```python
from build123d import *

# Parameters (mm, degrees)
F0_W     = 110
F0_H     = 55
F1_DEPTH = 60
F3_DEPTH = 60.001
F5_DEPTH = 35


with BuildPart() as f1:
    # F0 (on Top) → F1 (new body)
    with BuildSketch(Plane.XY):
        Rectangle(F0_W, F0_H)
    extrude(amount=F1_DEPTH)

    # F2 (on face) → F3 (cut, through all)
    with BuildSketch(Plane.XY.offset(60)):
        Polygon((-15, -27.5), (-55, 12.5), (-55, -27.5), align=None)
    extrude(amount=-F3_DEPTH, mode=Mode.SUBTRACT)

    # F4 (on face) → F5 (cut)
    with BuildSketch(Plane.XY.offset(60)):
        Polygon((-15, -27.5), (25, -27.5), (25, 12.5), (-15, 12.5), (-15, 27.5), (-55, 27.5), (-55, 12.5), align=None)
    extrude(amount=-F5_DEPTH, mode=Mode.SUBTRACT)


solid = f1.part
```
Design review of the part built by this model. Coordinates are the model's own, in mm. A direction names the side the tool comes from. Coordinates: 2 decimals unless noted, no trailing zeros. Order: outer loops, then holes, each group sorted by start corner. A loop starts at its lowest first (then second) coordinate and runs counter-clockwise, first axis right, second up. Notation, with made-up numbers: M 4,84 L 38,84 A11 cw 38,103 Z; hole C 70.25,48.25 d3. An arc over 180 degrees is marked long. Answer as a JSON object with one key per item and string values. Group by question number.
1) Add section A-A, the plane x = 10. Write out the cut boundary in (y, z).
2) Tool access review of faces 1 (the flat face through (25, -8, 43)), 2 (the flat face through (55, 0, 30)), 3 (the flat face through (-15, 20, 43)): name each direction out of +Z, -Z, +X, -X, +Y, -Y from which nothing blocks a thin tool from reaching the whole face with its end or side.
3) For pin 1 (3 mm diameter, centred on x = 0.5, z = 47, fed in from -Y); pin 2 (7.5 mm diameter, centred on y = 20.5, z = 50, fed in from -X); pin 3 (17.5 mm diameter, centred on y = 1, z = 36, fed in from -X), all flat-tipped, find the tip position at first contact; note any pin that passes through.
4) Add section B-B, the plane y = -24. Write out the cut boundary in (x, z), then the cut area to 3 significant figures.
5) Wall thickness on L1, parallel to X at y = 17, z = 26.5; L2, parallel to X at y = -7.5, z = 27.5; L3, parallel to Z at x = -22, y = 0: over which ranges is each line inside the solid? List them lowest first.
Computed values:
{
 "1": {"outline": "M -27.5,0 L 27.5,0 L 27.5,60 L 12.5,60 L 12.5,25 L -27.5,25 Z"},
 "2": {"face 1": "+Z, -X, -Y", "face 2": "+Z, -Z, +X, +Y, -Y", "face 3": "+Z, -X, +Y, -Y"},
 "3": {"pin 1": "stops at y = 12.5", "pin 2": "stops at x = -15", "pin 3": "stops at x = 25"},
 "4": {"outline": "M -18.5,0 L 55,0 L 55,60 L 25,60 L 25,25 L -18.5,25 Z", "area": "2,890 mm^2"},
 "5": {"L1": "x = -15 to 55", "L2": "x = 25 to 55", "L3": "z = 0 to 25"}
}
